Part model, mm, in its own coordinate system. Give positions to 0.01 mm unless a question says otherwise; leave off trailing zeros. Order: outer loops, then holes, each group sorted by start corner. A loop starts at its lowest first (then second) coordinate and runs counter-clockwise, first axis right, second up.
1. Drop a flat-ended pin along its axis: pin 1 Ø2.5 at (x, y) = (0, 67.5) entering from +Z. Give the stop position or say it passes through.
2. Slice it at A-A on z = 3.75. List the corners of the cut face in (x, y).
3. Probe line 1 (X direction, y = 156.25, z = -7.3); line 2 (X direction, y = 158.5, z = -0.25). List the from-to ranges inside material, lowest first.
4. Slice it at B-B on y = 122. List the corners of the cut face in (x, z), and give its area (3 significant figures).
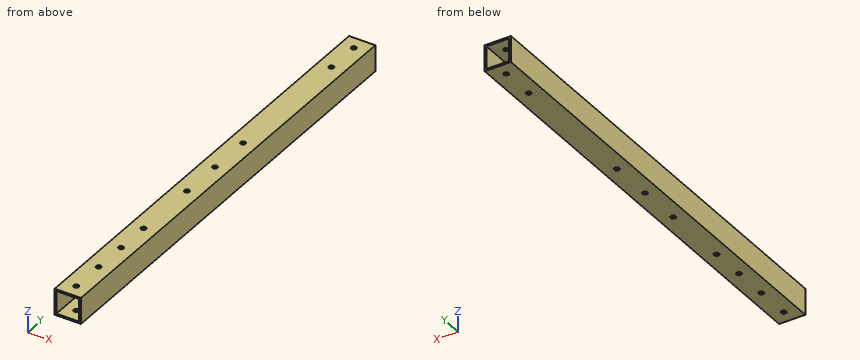
from build123d import *

# Parameters (mm, degrees)
SKETCH_1_W          = 15
SKETCH_1_H          = 15
SKETCH_1_W_2        = 13
SKETCH_1_H_2        = 13
EXTRUDE_1_DEPTH     = 262.5
SKETCH_2_R          = 1.45
CUT_EXTRUDE_1_DEPTH = 264.035168751


with BuildPart() as part:
    # 草图1 → 拉伸-薄壁1 (new body)
    with BuildSketch(Plane(origin=(0, 0, 0), x_dir=(1, 0, 0), z_dir=(0, 1, 0))):
        Rectangle(SKETCH_1_W, SKETCH_1_H)
        Rectangle(SKETCH_1_W_2, SKETCH_1_H_2, mode=Mode.SUBTRACT)
    extrude(amount=EXTRUDE_1_DEPTH)

    # 草图2 → 切除-拉伸1 (cut, through all)
    with BuildSketch(Plane.XY.offset(7.5)):
        with Locations((0, 7.5)):
            Circle(SKETCH_2_R)
        with Locations((0, 27.5)):
            Circle(SKETCH_2_R)
        with Locations(Location((0, 235, 0), (0, 0, 180))):
            Circle(SKETCH_2_R)
        with Locations(Location((0, 255, 0), (0, 0, 180))):
            Circle(SKETCH_2_R)
        with Locations((0, 131.25)):
            Circle(SKETCH_2_R)
        with Locations((0, 106.25)):
            Circle(SKETCH_2_R)
        with Locations((0, 156.25)):
            Circle(SKETCH_2_R)
        with Locations((0, 47.5)):
            Circle(SKETCH_2_R)
        with Locations((0, 67.5)):
            Circle(SKETCH_2_R)
    extrude(amount=-CUT_EXTRUDE_1_DEPTH, mode=Mode.SUBTRACT)


solid = part.part
Data:
1. pin 1: passes through
2. outline: (-7.5, 0) - (-6.5, 0) - (-6.5, 262.5) - (-7.5, 262.5) - close; (6.5, 0) - (7.5, 0) - (7.5, 262.5) - (6.5, 262.5) - close
3. line 1: x = -7.5 to -1.45, 1.45 to 7.5
3. line 2: x = -7.5 to -6.5, 6.5 to 7.5
4. outline: (-7.5, -7.5) - (7.5, -7.5) - (7.5, 7.5) - (-7.5, 7.5) - close; hole (-6.5, -6.5) - (6.5, -6.5) - (6.5, 6.5) - (-6.5, 6.5) - close
4. area: 56.0 mm2
